```python
from build123d import *

# Parameters (mm, degrees)
F0_R     = 1.5
F1_DEPTH = 1.25


with BuildPart() as f1:
    # F0 (on Front) → F1 (new body, symmetric)
    with BuildSketch(Plane.XZ):
        Polygon((0, 0), (50, 0), (50, 3), (3.419785, 3.088514), (3.511779, 51.5), (-14.488221, 51.5), (-14.488221, 21.658587), (-8.945253, 15), (0, 15), align=None)
        with Locations((-8, 20)):
            Circle(F0_R, mode=Mode.SUBTRACT)
        with Locations((-11.488221, 46.5)):
            Circle(F0_R, mode=Mode.SUBTRACT)
    extrude(amount=F1_DEPTH, both=True)


solid = f1.part
```
Design review of the part built by this model. Coordinates are the model's own, in mm. A direction names the side the tool comes from. Coordinates: 2 decimals unless noted, no trailing zeros. Order: outer loops, then holes, each group sorted by start corner. A loop starts at its lowest first (then second) coordinate and runs counter-clockwise, first axis right, second up.
1) Clearance check with a flat-ended pin moving along its axis: pin 1 (1.2 mm diameter, centred on x = -4.5, y = -0.5, fed in from -Z). State where the tip first meets the part, or that it passes through.
2) Take a section at D-D, the plane z = 36.5. Give the boundary of the cut face in (x, y).
3) Take a section at B-B, the plane z = 20. Give the boundary of the cut face in (x, y), and give its area (3 significant figures).
4) Take a section at A-A, the plane x = -8. Give the boundary of the cut face in (y, z), and give its area (4 significant figures).
5) For faces 5 (the flat face through (50, 0, 1)), 6 (the flat face through (0, 0, 8)), list the 3-axis set-ups (+Z, -Z, +X, -X, +Y, -Y) from which the entire face can be reached by the end or side of a thin tool; tool diameter is ignored.
6) Take a section at C-C, the plane y = -0.5. Give the boundary of the cut face in (x, z).
7) Mouldability with a two-part tool opening along Z and no side actions: class faces 1 (the flat face through (1, -1.25, 24)), 2 (the flat face through (25, 0, 0)), 3 (the cylindrical face through (-11.813, 0.018, 45.036)), 4 (the flat face through (-5, 0, 51.5)) as +Z half, -Z half, draft (parallel to the pull), parting line (faces both ways), or undercut.
8) Wall thickness on line 1 along Z through (x, y) = (-8, 0.4); line 2 along Z through (x, y) = (47.5, 0.95); line 3 along Z through (x, y) = (11, 0.1): over which ranges is each line inside the solid? List them lowest first.
Returned:
1. pin 1: stops at z = 15
2. outline: (-14.49, -1.25) - (3.48, -1.25) - (3.48, 1.25) - (-14.49, 1.25) - close
3. outline: (-13.11, -1.25) - (-9.5, -1.25) - (-9.5, 1.25) - (-13.11, 1.25) - close; (-6.5, -1.25) - (3.45, -1.25) - (3.45, 1.25) - (-6.5, 1.25) - close
3. area: 33.9 mm2
4. outline: (-1.25, 15) - (1.25, 15) - (1.25, 18.5) - (-1.25, 18.5) - close; (-1.25, 21.5) - (1.25, 21.5) - (1.25, 51.5) - (-1.25, 51.5) - close
4. area: 83.75 mm2
5. face 5: +Z, -Z, +X, +Y, -Y
5. face 6: -Z, -X, +Y, -Y
6. outline: (-14.49, 21.66) - (-8.95, 15) - (0, 15) - (0, 0) - (50, 0) - (50, 3) - (3.42, 3.09) - (3.51, 51.5) - (-14.49, 51.5) - close; hole circle Ø3 at (-11.49, 46.5); hole circle Ø3 at (-8, 20)
7. face 1: draft
7. face 2: -Z half
7. face 3: undercut
7. face 4: +Z half
8. line 1: z = 15 to 18.5, 21.5 to 51.5
8. line 2: z = 0 to 3
8. line 3: z = 0 to 3.07
